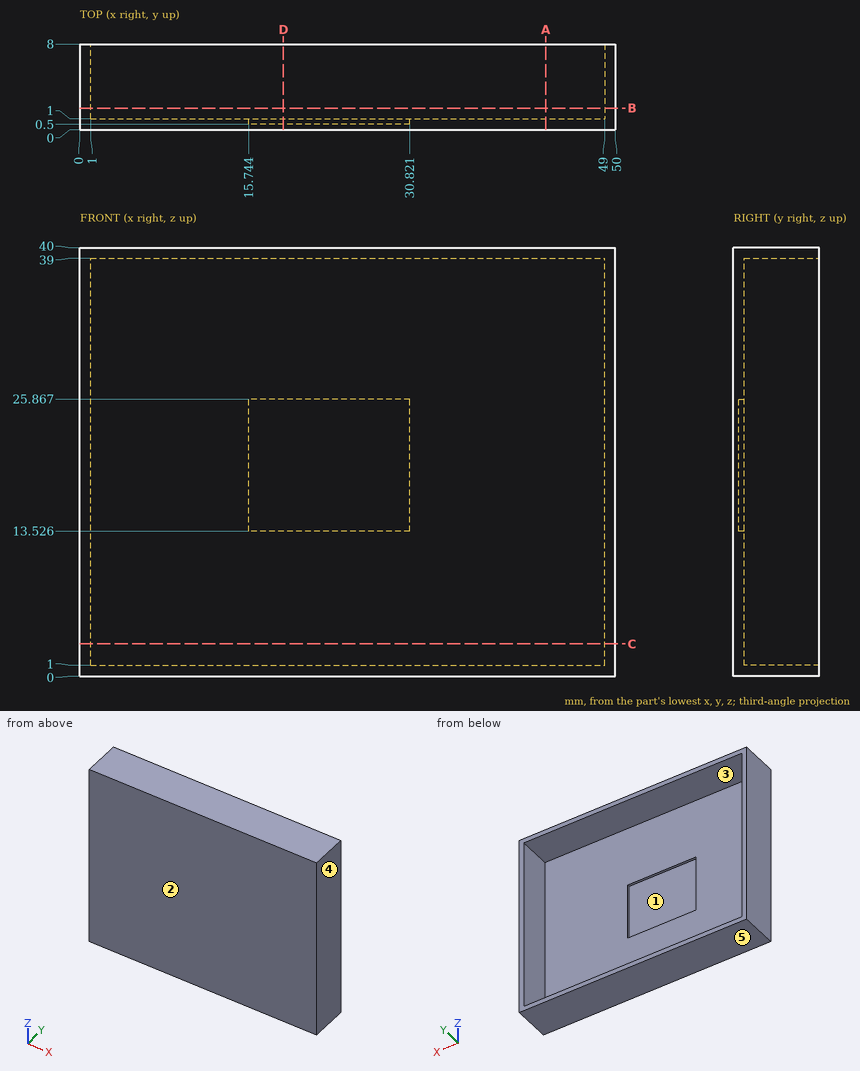
Input: dimensioned drawing with shaded views. Units: mm. Origin: part minimum x, y, z. A direction names the side the tool comes from. Give positions to 0.01 mm unless a question says otherwise; leave off trailing zeros. Write each loop counter-clockwise with the first axis right and the second up, starting at its lowest first coordinate (ties: lowest second). Pieces come first, ordered by that corner, then holes.
1. Material intervals for line 1 along Z through (x, y) = (11, 5.25); line 2 along X through (y, z) = (7, 5); line 3 along Y through (x, z) = (30, 6), sorted ascending.
2. Section query B-B (y = 2). Return the cut outline in (x, z).
3. Access query for the marked faces 1 and 2. Directions: +Z, -Z, +X, -X, +Y, -Y. A direction counts if a zero-diameter tool reaches every point of the face in a straight line with its end or side. Return the directions, or none.
4. Section query A-A (x = 43.5). Return the cut outline in (y, z).
5. Section query C-C (z = 3). Return the cut outline in (x, y).
6. Pull-direction query (X, two-part tool) for the marked faces 3, 4 and 5; classes: +X half, -X half, draft (parallel to the pull), parting line (faces both ways), or undercut.
7. First-contact query: pin 1 (13.5 mm diameter, centred on x = 24, z = 21, fed in from +Y). Flat tip, straight axial feed; report the tip coordinate or a pass-through.
8. Section query D-D (x = 19). Return the cut outline in (y, z).
Output values:
1. line 1: z = 0 to 1, 39 to 40
1. line 2: x = 0 to 1, 49 to 50
1. line 3: y = 0 to 1
2. outline: (0, 0) - (50, 0) - (50, 40) - (0, 40) - close; hole (1, 1) - (49, 1) - (49, 39) - (1, 39) - close
3. face 1: +Y
3. face 2: +Z, -Z, +X, -X, -Y
4. outline: (0, 0) - (8, 0) - (8, 1) - (1, 1) - (1, 39) - (8, 39) - (8, 40) - (0, 40) - close
5. outline: (0, 0) - (50, 0) - (50, 8) - (49, 8) - (49, 1) - (1, 1) - (1, 8) - (0, 8) - close
6. face 3: undercut
6. face 4: +X half
6. face 5: draft
7. pin 1: stops at y = 1
8. outline: (0, 0) - (8, 0) - (8, 1) - (1, 1) - (1, 13.53) - (0.5, 13.53) - (0.5, 25.87) - (1, 25.87) - (1, 39) - (8, 39) - (8, 40) - (0, 40) - close
